```python
from build123d import *

# Parameters (mm, degrees)
SKETCH1_W            = 84
SKETCH1_H            = 84
BOSS_EXTRUDE1_DEPTH  = 6
SKETCH2_R            = 1.5
CUT_EXTRUDE1_DEPTH   = 6
LPATTERN1_COUNT      = 2
LPATTERN1_PITCH      = 72
LPATTERN1_COUNT_DIR2 = 2
LPATTERN1_PITCH_DIR2 = 60
SKETCH3_R            = 1.549904247
SKETCH3_R_2          = 1.748244363
CUT_EXTRUDE2_DEPTH   = 10


with BuildPart() as part:
    # Sketch1 → Boss-Extrude1 (new body)
    with BuildSketch(Plane(origin=(0, 0, 0), x_dir=(1, 0, 0), z_dir=(0, 1, 0))):
        with Locations((42, 42)):
            Rectangle(SKETCH1_W, SKETCH1_H)
    extrude(amount=BOSS_EXTRUDE1_DEPTH)

    # Sketch2 → Cut-Extrude1 (cut)
    with BuildSketch(Plane(origin=(0, 6, 0), x_dir=(1, 0, 0), z_dir=(0, 1, 0))):
        with Locations(Location((6, 72, 0), (0, 0, 270))):
            Circle(SKETCH2_R)
    cut_extrude1 = extrude(amount=-CUT_EXTRUDE1_DEPTH, mode=Mode.SUBTRACT)

    # LPattern1: Cut-Extrude1 2 × 2
    with Locations(*[(i * LPATTERN1_PITCH, 0, j * LPATTERN1_PITCH_DIR2) for i in range(LPATTERN1_COUNT) for j in range(LPATTERN1_COUNT_DIR2) if (i, j) != (0, 0)]):
        add(cut_extrude1, mode=Mode.SUBTRACT)

    # Sketch3 → Cut-Extrude2 (cut)
    with BuildSketch(Plane.ZY):
        with Locations((-81, 3)):
            Circle(SKETCH3_R)
        with Locations((-3, 3)):
            Circle(SKETCH3_R_2)
    cut_extrude2 = extrude(amount=-CUT_EXTRUDE2_DEPTH, mode=Mode.SUBTRACT)

    # Mirror1: Cut-Extrude2 across plane
    add(cut_extrude2.mirror(Plane.ZY.offset(-42)), mode=Mode.SUBTRACT)


solid = part.part
```
CAD build for the part. Positions are in the model's coordinates, mm. A direction names the side the tool comes from. Give positions to 0.01 mm unless a question says otherwise; leave off trailing zeros. Write each loop counter-clockwise with the first axis right and the second up, starting at its lowest first coordinate (ties: lowest second). Pieces come first, ordered by that corner, then holes. Notation, with made-up numbers: M -34,37.5 L -15,37.5 A4 ccw -15,42.5 Z; hole C 36,80.25 d5. An arc over 180 degrees is marked long. Return JSON: item names as keys, results as strings. Group by question number.
(1) Band-saw the part on D-D (z = -72). Give the cut face in (x, y), and give its area (3 significant figures).
(2) Mould opens along Z. For faces 1 (the face through (41, 3, 0)), 2 (the face through (41, 3, -84)), 3 (the face through (74, 3, -81)), 4 (the face through (41, 0, -43)) say: pulls with the +Z half, pulls with the -Z half, needs draft (parallel to the pull), parting line crosses it, or undercut.
(3) Band-saw the part on C-C (z = -81). Give the cut face in (x, y), and give its area (3 significant figures).
(4) Drill centre lines: L1, parallel to Y at x = 7.25, z = -3; L2, parallel to X at y = 5.65, z = -12; L3, parallel to Y at x = 5.75, z = -81. Where is each one in solid material? Low to high. Write a range as [from, to].
(5) Flat gauge pins, fed straight in: pin 1 Ø1 at (y, z) = (3, -4) entering from -X; pin 2 Ø1.5 at (y, z) = (2.5, -81) entering from +X. Where does each tip first touch, or does it go through?
(6) 3-axis set-ups, long thin cutter, end or side, ignore diameter. For faces 5 (the face through (4.93, 3.07, -82.55)), 6 (the face through (6.45, 3.04, -70.57)), 7 (the face through (79.07, 3.07, -82.55)): which of +Z, -Z, +X, -X, +Y, -Y reach the whole face in a straight line?
(7) Band-saw the part on B-B (y = 3). Give the cut face in (x, z).
(8) Band-saw the part on A-A (x = 78). Give the cut face in (y, z), and give its area (3 significant figures).
Entries:
{
 "1": {"outline": "M 0,0 L 4.5,0 L 4.5,6 L 0,6 Z; M 7.5,0 L 76.5,0 L 76.5,6 L 7.5,6 Z; M 79.5,0 L 84,0 L 84,6 L 79.5,6 Z", "area": "468 mm^2"},
 "2": {"face 1": "pulls with the +Z half", "face 2": "pulls with the -Z half", "face 3": "undercut", "face 4": "needs draft"},
 "3": {"outline": "M 0,0 L 84,0 L 84,1.45 L 74,1.45 L 74,4.55 L 84,4.55 L 84,6 L 0,6 L 0,4.55 L 10,4.55 L 10,1.45 L 0,1.45 Z", "area": "442 mm^2"},
 "4": {"L1": "y = [0, 1.25], [4.75, 6]", "L2": "x = [0, 4.5], [7.5, 76.5], [79.5, 84]", "L3": "y = [0, 1.45], [4.55, 6]"},
 "5": {"pin 1": "stops at x = 10", "pin 2": "stops at x = 74"},
 "6": {"face 5": "-X", "face 6": "+Y, -Y", "face 7": "+X"},
 "7": {"outline": "M 0,-84 L 84,-84 L 84,-82.55 L 74,-82.55 L 74,-79.45 L 84,-79.45 L 84,-4.75 L 74,-4.75 L 74,-1.25 L 84,-1.25 L 84,0 L 0,0 L 0,-1.25 L 10,-1.25 L 10,-4.75 L 0,-4.75 L 0,-79.45 L 10,-79.45 L 10,-82.55 L 0,-82.55 Z; hole C 6,-72 d3; hole C 6,-12 d3; hole C 78,-72 d3; hole C 78,-12 d3"},
 "8": {"outline": "M 0,-84 L 6,-84 L 6,-73.5 L 0,-73.5 Z; M 0,-70.5 L 6,-70.5 L 6,-13.5 L 0,-13.5 Z; M 0,-10.5 L 6,-10.5 L 6,0 L 0,0 Z; hole C 3,-3 d3.5; hole C 3,-81 d3.1", "area": "451 mm^2"}
}
